Can you work these out from the drawing? Everything is in mm from the part's minimum corner. Coordinates: 2 decimals unless noted, no trailing zeros. Order: outer loops, then holes, each group sorted by start corner. A loop starts at its lowest first (then second) coordinate and runs counter-clockwise, first axis right, second up. Notation, with made-up numbers: (63, -20.5) -> (96, -20.5) arc R16 ccw to (96, -15.5) -> close; hole circle Ø4 at (-30.5, -24). An arc over 180 degrees is marked (long way). Return JSON: item names as keys, results as strings. Group by question number.
1) If I drill on probe 1 along Y at (x, z) = (202, 9); probe 2 along Z at (x, y) = (190, 66) (3 decimals); probe 3 along X at (y, z) = (92, 9), over which ranges is the centre line in solid material (lowest first)? Write a range as from..to.
2) If we section it at A-A, the plane x = 410.5: Please give me the cut outline in (y, z) (3 decimals).
3) If we section it at B-B, the plane y = 62: Please give me the cut outline in (x, z) (3 decimals).
4) For pin 1 (9.5 mm diameter, centred on x = 292, y = 58.5, fed in from -Z) (3 decimals), with a flat end and sliding along its axis, tell me the tip position at first contact or that it passes through.
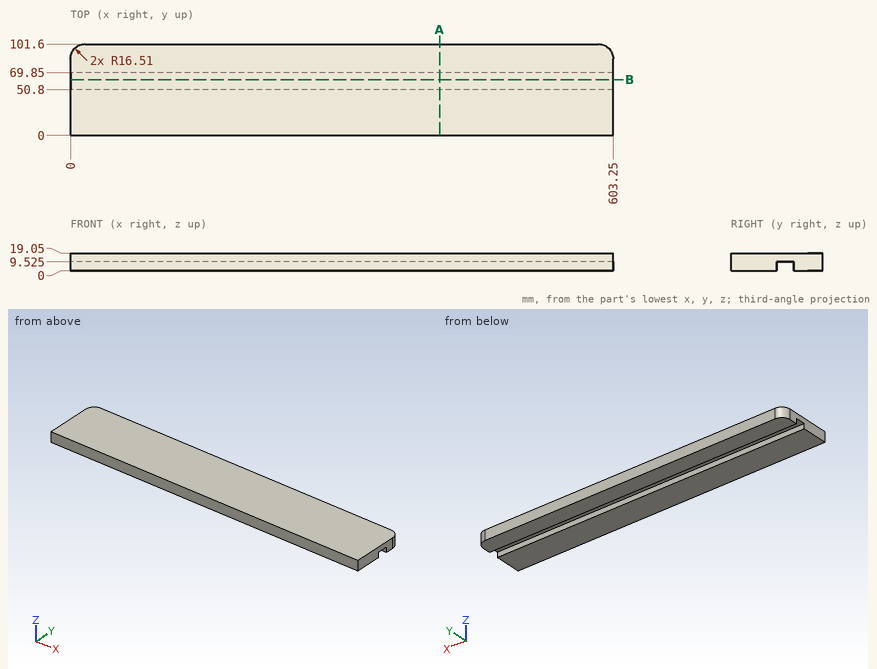
Result sheet:
{
 "1": {"probe 1": "y = 0..50.8, 69.85..101.6", "probe 2": "z = 9.525..19.05", "probe 3": "x = 1.52..601.73"},
 "2": {"outline": "(0, 0) -> (50.8, 0) -> (50.8, 9.525) -> (69.85, 9.525) -> (69.85, 0) -> (101.6, 0) -> (101.6, 19.05) -> (0, 19.05) -> close"},
 "3": {"outline": "(0, 9.525) -> (603.25, 9.525) -> (603.25, 19.05) -> (0, 19.05) -> close"},
 "4": {"pin 1": "stops at z = 9.525"}
}
